from build123d import *

# Parameters (mm, degrees)
SKETCH1_R           = 6.5
BOSS_EXTRUDE1_DEPTH = 20
SKETCH2_R           = 4
CUT_EXTRUDE1_DEPTH  = 16
SKETCH3_R           = 2
CUT_EXTRUDE2_DEPTH  = 5
SKETCH4_R           = 10.5
SKETCH4_R_2         = 6.5
BOSS_EXTRUDE2_DEPTH = 2


with BuildPart() as part:
    # Sketch1 → Boss-Extrude1 (new body)
    with BuildSketch(Plane(origin=(0, 0, 0), x_dir=(1, 0, 0), z_dir=(0, 1, 0))):
        Circle(SKETCH1_R)
    extrude(amount=BOSS_EXTRUDE1_DEPTH)

    # Sketch2 → Cut-Extrude1 (cut)
    with BuildSketch(Plane(origin=(0, 20, 0), x_dir=(1, 0, 0), z_dir=(0, 1, 0))):
        Circle(SKETCH2_R)
    extrude(amount=-CUT_EXTRUDE1_DEPTH, mode=Mode.SUBTRACT)

    # Sketch3 → Cut-Extrude2 (cut, through all)
    with BuildSketch(Plane(origin=(0, 4, 0), x_dir=(1, 0, 0), z_dir=(0, 1, 0))):
        Circle(SKETCH3_R)
    extrude(amount=-CUT_EXTRUDE2_DEPTH, mode=Mode.SUBTRACT)

    # Sketch4 → Boss-Extrude2 (add)
    with BuildSketch(Plane(origin=(0, 20, 0), x_dir=(1, 0, 0), z_dir=(0, 1, 0))):
        Circle(SKETCH4_R)
        Circle(SKETCH4_R_2, mode=Mode.SUBTRACT)
    extrude(amount=-BOSS_EXTRUDE2_DEPTH)


solid = part.part
Verification items for the finished model (mm, model axes). A direction names the side the tool comes from. Give positions to 0.01 mm unless a question says otherwise; leave off trailing zeros. Order: outer loops, then holes, each group sorted by start corner. A loop starts at its lowest first (then second) coordinate and runs counter-clockwise, first axis right, second up. Notation, with made-up numbers: M -13,30 L 28,30 A14 ccw 28,49 Z; hole C 8.5,-8.5 d7. An arc over 180 degrees is marked long. Use one line per item in the form item = value. Start each with the question number.
Q1. Section check B-B (x = 0). Enter the section's corners in (y, z), then the cut area to 3 significant figures.
Q2. Access from +Z, -Z, +X, -X, +Y, -Y to the whole of each face (thin tool, end or side, straight path). Record for faces 4 (the flat face through (1, 0, -2)), 5 (the flat face through (5, 18, -5)), 6 (the cylindrical face through (-0.867, 12.112, 3.905)).
Q3. Go/stop test with flat-tipped pins: pin 1 Ø10 at (x, y) = (-6, 10) entering from +Z; pin 2 Ø4 at (y, z) = (12, 6.5) entering from -X; pin 3 Ø4 at (x, z) = (8, -3.5) entering from -Y. Record where each tip stops, or that it passes through.
Q4. Section check C-C (y = 10.25). Enter the section's corners in (x, z), then the cut area to 3 significant figures.
Q5. Section check A-A (z = 0). Enter the section's corners in (x, y).
Q6. Scan lines: line 1 along Z through (x, y) = (0, 1); line 2 along X through (y, z) = (9, 0). Record each from-to range of solid material in increasing order. Write a range as [from, to].
Q7. Mould release check, pull along X, two halves, no side actions. Record for faces 1 (the flat face through (5, 20, 0)), 2 (the cylindrical face through (-5.158, 8.874, 3.955)), 3 (the flat face through (-2, 4, 1)): +X half, -X half, draft (parallel to the pull), parting line (faces both ways), or undercut.
Q8. Section check D-D (x = 2.5). Enter the section's corners in (y, z), then the cut area to 3 significant figures.
Evaluation:
q1.outline = M 0,-6.5 L 18,-6.5 L 18,-10.5 L 20,-10.5 L 20,-4 L 4,-4 L 4,-2 L 0,-2 Z; M 0,2 L 4,2 L 4,4 L 20,4 L 20,10.5 L 18,10.5 L 18,6.5 L 0,6.5 Z
q1.area = 132 mm2
q2.face_4 = +Z, -Z, +X, -X, -Y
q2.face_5 = -Y
q2.face_6 = +Y
q3.pin_1 = 6.42
q3.pin_2 = -4.69
q3.pin_3 = 18
q4.outline = C 0,0 d13; hole C 0,0 d8
q4.area = 82.5 mm2
q5.outline = M -10.5,18 L -6.5,18 L -6.5,0 L -2,0 L -2,4 L -4,4 L -4,20 L -10.5,20 Z; M 2,0 L 6.5,0 L 6.5,18 L 10.5,18 L 10.5,20 L 4,20 L 4,4 L 2,4 Z
q6.line_1 = [-6.5, -2], [2, 6.5]
q6.line_2 = [-6.5, -4], [4, 6.5]
q7.face_1 = draft
q7.face_2 = parting line
q7.face_3 = undercut
q8.outline = M 0,-6 L 18,-6 L 18,-10.2 L 20,-10.2 L 20,-3.12 L 4,-3.12 L 4,3.12 L 20,3.12 L 20,10.2 L 18,10.2 L 18,6 L 0,6 Z
q8.area = 157 mm2
